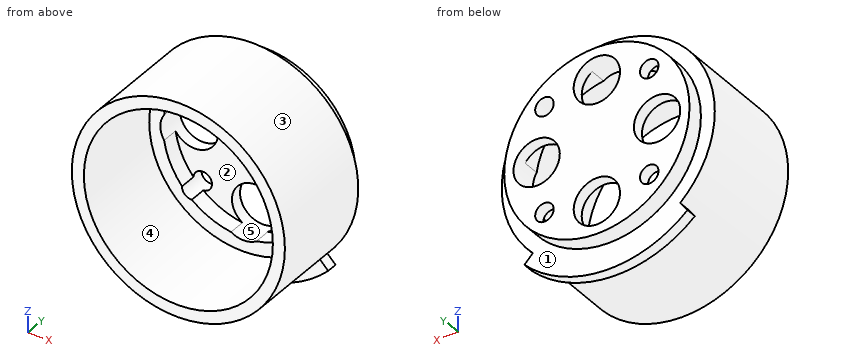
Autodesk Inventor part; units mm, degrees
ref_plane "XZ Plane" through (0, 0, 0) normal (0, 1, 0) x (-1, 0, 0)
sketch "Sketch1" plane through (0, 0, 0) normal (0, 1, 0) x (-1, 0, 0)
  circle A0 centre (0, 0) radius 11.5
  dimension "d0" = 23
extrude "Extrusion1" add sketch "Sketch1" along normal blind 11.9
sketch "Sketch2" plane through (0, 11.9, 0) normal (0, 1, 0) x (1, 0, 0)
  circle A0 centre (0, 0) radius 10
  dimension "d3" = 20
extrude "Extrusion2" add sketch "Sketch2" along normal blind 1.85
sketch "Sketch3" plane through (0, 13.75, 0) normal (0, 1, 0) x (1, 0, 0)
  circle A0 centre (0, 0) radius 10
  circle A1 centre (0, 6.5) radius 2.5
  dimension "d6" = 5
  dimension "d23" = 6.5
extrude "Extrusion3" cut sketch "Sketch3" against normal blind 5 contours A1
ref_plane "Work Plane1" through (0, 0, 0) normal (0.7071068, 0, 0.7071068) x (0, 1, 0)
sketch "Sketch4" plane through (0, 13.75, 0) normal (0, 1, 0) x (1, 0, 0)
  line L0 (16.1, 16.1) -> (-16.1, -16.1)
  point P0 (0, 0)
  point P1 (5.6569, 5.6569)
  dimension "d10" = 8
hole "Hole1" at (5.6569, 13.75, -5.6569) direction (0, -1, 0) diameter 2 depth 4.5 tip angle 118
pattern_circular "Circular Pattern1" count 4 over 360 about axis through (0, -10, 0) along (0, 1, 0) of "Extrusion3", "Hole1"
shell "Shell1" thickness 1.3 removed faces 17 at (-0.1507, 0, 2.542) at (-0.852, 8.75, -7.0526) at (6.099, 10.4167, 2.4676) at (7.0526, 8.75, -0.852) at (2.4676, 10.4167, -6.099) at (5.7373, 12.25, -4.6601) at (5.843, 9.1165, -4.9017) at (6.3455, 9.1165, 6.0183) at (4.6601, 12.25, 5.7373) at (0.852, 8.75, 7.0526) at (-2.4676, 10.4167, 6.099) at (-7.0526, 8.75, 0.852) at (-6.099, 10.4167, -2.4676) at (-5.843, 9.1165, 4.9017) at (-5.7373, 12.25, 4.6601) at (-4.9017, 9.1165, -5.843) at (-4.6601, 12.25, -5.7373)
sketch "Sketch5" plane through (0, 11.9, 0) normal (0, 1, 0) x (1, 0, 0)
  arc A0 (9.0498, 9.0605) -> (-8.5529, 9.531) centre (0, 0) ccw
  arc A1 (8.1423, 8.1211) -> (-7.76, 8.4872) centre (0, 0) ccw
  line L0 (-8.5529, 9.531) -> (-7.76, 8.4872)
  line L1 (8.1423, 8.1211) -> (9.0498, 9.0605)
extrude "Extrusion4" add sketch "Sketch5" against normal blind 1.2
properties part number "motor_GM1806-80T_SkyproRO_stator" material "Iron, Cast"
For this review, take the finished solid that the model builds, in its own axes (mm). Face numbers are marked on the shaded views. A direction names the side the tool comes from. Coordinates: 2 decimals unless noted, no trailing zeros. Loops run counter-clockwise (first coordinate to the right, second up) from the corner with the lowest first, then second, coordinate; pieces in that order, holes last. Notation, with made-up numbers: (53, 59) -> (88, 59) arc R15 cw to (88, 81) -> close; hole circle Ø9 at (-10.5, 24). An arc over 180 degrees is marked (long way). Return JSON: item names as keys, results as strings. Group by question number.
(1) Consider section C-C, the plane x = -9.5. Give the boundary of the cut face in (y, z), plus the area to 3 significant figures.
(2) Consider section A-A, the plane x = 2. Give the boundary of the cut face in (y, z).
(3) Mouldability with a two-part tool opening along X and no side actions: class the marked faces 1, 2 and 3 as pulls with the +X half, pulls with the -X half, needs draft (parallel to the pull), parting line crosses it, or undercut.
(4) For pin 1 Ø6 at (x, y) = (-5.5, 9.5) entering from +Z (3 decimals); pin 2 Ø1 at (y, z) = (9.5, -3) entering from -X (3 decimals); pin 3 Ø8.5 at (x, z) = (-4, 3.5) entering from -Y, all flat-tipped, find the tip position at first contact; note any pin that passes through.
(5) Consider section B-B, the plane y = 5.25. Give the boundary of the cut face in (x, z).
(6) Tool access review of the marked faces 4 and 5: name each direction out of +Z, -Z, +X, -X, +Y, -Y from which nothing blocks a thin tool from reaching the whole face with its end or side.
(7) To check wall thickness, follow L1, parallel to X at y = 11.3, z = 0; L2, parallel to Y at x = -0.75, z = -1; L3, parallel to Z at x = 7.25, y = 1.5. State the ranges of each line that lie inside material, in increasing order.
Results below:
{
 "1": {"outline": "(0, -6.48) -> (11.9, -6.48) -> (11.9, -3.12) -> (13.75, -3.12) -> (13.75, 3.12) -> (11.9, 3.12) -> (11.9, 6.48) -> (0, 6.48) -> (0, 3.71) -> (10.6, 3.71) -> (10.6, -3.71) -> (0, -3.71) -> close", "area": "87.1 mm2"},
 "2": {"outline": "(0, -11.32) -> (10.7, -11.32) -> (10.7, -12.65) -> (11.9, -12.65) -> (11.9, -9.8) -> (13.75, -9.8) -> (13.75, -8) -> (12.45, -8) -> (12.45, -8.47) -> (10.6, -8.47) -> (10.6, -10) -> (0, -10) -> close; (0, 10) -> (10.6, 10) -> (10.6, 8.47) -> (12.45, 8.47) -> (12.45, 8) -> (13.75, 8) -> (13.75, 9.8) -> (11.9, 9.8) -> (11.9, 11.32) -> (0, 11.32) -> close; (12.45, -5) -> (13.75, -5) -> (13.75, 5) -> (12.45, 5) -> close"},
 "3": {"face 1": "needs draft", "face 2": "undercut", "face 3": "parting line crosses it"},
 "4": {"pin 1": "stops at z = 11.225", "pin 2": "stops at x = -11.225", "pin 3": "stops at y = 10.6"},
 "5": {"outline": "circle Ø23 at (0, 0); hole circle Ø20.4 at (0, 0)"},
 "6": {"face 4": "-Y", "face 5": "+Y, -Y"},
 "7": {"L1": "x = -11.5 to -9, 9 to 11.5", "L2": "y = 12.45 to 13.75", "L3": "z = -8.93 to -7.17, 7.17 to 8.93"}
}
